Work out the finished part from the listing and answer in its coordinate system (mm). A direction names the side the tool comes from. Round coordinates to 2 decimals unless told otherwise and drop trailing zeros. Loops run counter-clockwise (first coordinate to the right, second up) from the corner with the lowest first, then second, coordinate; pieces in that order, holes last. Notation, with made-up numbers: M -12,76 L 8,76 A13 ccw 8,95 Z; hole C 43,33 d9. An arc over 180 degrees is marked long. One line per item, written item: value.
```python
from build123d import *

# Parameters (mm, degrees)
BOSS_EXTRUDE1_DEPTH = 6.35
CUT_EXTRUDE1_DEPTH  = 7.35
SKETCH3_R           = 2.286
CUT_EXTRUDE2_DEPTH  = 7.35
BOSS_EXTRUDE2_DEPTH = 6.35
SKETCH5_R           = 4.826
BOSS_EXTRUDE3_DEPTH = 6.35
SKETCH6_R           = 2.286
CUT_EXTRUDE3_DEPTH  = 13.7


with BuildPart() as part:
    # Sketch1 → Boss-Extrude1 (new body)
    with BuildSketch(Plane(origin=(0, 0, 0), x_dir=(1, 0, 0), z_dir=(0, 1, 0))):
        Polygon((0, 192.024), (6.35, 198.374), (196.85, 198.374), (203.2, 192.024), (203.2, 6.35), (196.85, 0), (6.35, 0), (0, 6.35), align=None)
    extrude(amount=BOSS_EXTRUDE1_DEPTH)

    # Sketch2 → Cut-Extrude1 (cut, through all)
    with BuildSketch(Plane(origin=(0, 6.35, 0), x_dir=(1, 0, 0), z_dir=(0, 1, 0))):
        with BuildLine():
            Line((45.682614691, 180.594), (152.691385309, 180.594))
            ThreePointArc((152.691385309, 180.594), (158.558020341, 176.674039796), (157.18151337, 169.753871939))
            Line((157.18151337, 169.753871939), (103.677128061, 116.24948663))
            ThreePointArc((103.677128061, 116.24948663), (99.187, 114.389614691), (94.696871939, 116.24948663))
            Line((94.696871939, 116.24948663), (41.19248663, 169.753871939))
            ThreePointArc((41.19248663, 169.753871939), (39.815979659, 176.674039796), (45.682614691, 180.594))
        make_face()
        with BuildLine():
            Line((17.78, 152.691385309), (17.78, 45.682614691))
            ThreePointArc((17.78, 45.682614691), (21.699960204, 39.815979659), (28.620128061, 41.19248663))
            Line((28.620128061, 41.19248663), (82.12451337, 94.696871939))
            ThreePointArc((82.12451337, 94.696871939), (83.984385309, 99.187), (82.12451337, 103.677128061))
            Line((82.12451337, 103.677128061), (28.620128061, 157.18151337))
            ThreePointArc((28.620128061, 157.18151337), (21.699960204, 158.558020341), (17.78, 152.691385309))
        make_face()
        with BuildLine():
            Line((45.682614691, 17.78), (152.691385309, 17.78))
            ThreePointArc((152.691385309, 17.78), (158.558020341, 21.699960204), (157.18151337, 28.620128061))
            Line((157.18151337, 28.620128061), (103.677128061, 82.12451337))
            ThreePointArc((103.677128061, 82.12451337), (99.187, 83.984385309), (94.696871939, 82.12451337))
            Line((94.696871939, 82.12451337), (41.19248663, 28.620128061))
            ThreePointArc((41.19248663, 28.620128061), (39.815979659, 21.699960204), (45.682614691, 17.78))
        make_face()
        with BuildLine():
            Line((185.42, 157.517385309), (185.42, 40.856614691))
            ThreePointArc((185.42, 40.856614691), (181.500039796, 34.989979659), (174.579871939, 36.36648663))
            Line((174.579871939, 36.36648663), (116.24948663, 94.696871939))
            ThreePointArc((116.24948663, 94.696871939), (114.389614691, 99.187), (116.24948663, 103.677128061))
            Line((116.24948663, 103.677128061), (174.579871939, 162.00751337))
            ThreePointArc((174.579871939, 162.00751337), (181.500039796, 163.384020341), (185.42, 157.517385309))
        make_face()
    extrude(amount=-CUT_EXTRUDE1_DEPTH, mode=Mode.SUBTRACT)

    # Sketch3 → Cut-Extrude2 (cut, through all)
    with BuildSketch(Plane(origin=(0, 6.35, 0), x_dir=(1, 0, 0), z_dir=(0, 1, 0))):
        with Locations((11.73734, 11.73734)):
            Circle(SKETCH3_R)
        with Locations((191.46266, 11.73734)):
            Circle(SKETCH3_R)
        with Locations((191.46266, 186.63666)):
            Circle(SKETCH3_R)
        with Locations((11.73734, 186.63666)):
            Circle(SKETCH3_R)
    extrude(amount=-CUT_EXTRUDE2_DEPTH, mode=Mode.SUBTRACT)

    # Sketch4 → Boss-Extrude2 (add)
    with BuildSketch(Plane(origin=(0, 6.35, 0), x_dir=(1, 0, 0), z_dir=(0, 1, 0))):
        with BuildLine():
            Line((111.554726315, 180.594), (91.645273685, 180.594))
            ThreePointArc((91.645273685, 180.594), (94.961453031, 179.659298195), (97.301368182, 177.130363636))
            ThreePointArc((97.301368182, 177.130363636), (101.6, 174.498), (105.898631818, 177.130363636))
            ThreePointArc((105.898631818, 177.130363636), (108.238546969, 179.659298195), (111.554726315, 180.594))
        make_face()
    extrude(amount=-BOSS_EXTRUDE2_DEPTH)

    # Sketch5 → Boss-Extrude3 (add)
    with BuildSketch(Plane.XZ):
        with Locations((101.6, -179.324)):
            Circle(SKETCH5_R)
    extrude(amount=BOSS_EXTRUDE3_DEPTH)

    # Sketch6 → Cut-Extrude3 (cut, through all)
    with BuildSketch(Plane.XZ.offset(6.35)):
        with Locations((101.6, -179.324)):
            Circle(SKETCH6_R)
        with Locations((92.71, -184.404)):
            Circle(SKETCH6_R)
        with Locations((110.49, -184.404)):
            Circle(SKETCH6_R)
    extrude(amount=-CUT_EXTRUDE3_DEPTH, mode=Mode.SUBTRACT)


solid = part.part
```
1) Find section B-B (x = 66). Give the vertices of the cut face in (y, z), then the cut area to 3 significant figures.
Check values:
outline: M 0,-198.37 L 6.35,-198.37 L 6.35,-180.59 L 0,-180.59 Z; M 0,-144.95 L 6.35,-144.95 L 6.35,-119.8 L 0,-119.8 Z; M 0,-78.57 L 6.35,-78.57 L 6.35,-53.43 L 0,-53.43 Z; M 0,-17.78 L 6.35,-17.78 L 6.35,0 L 0,0 Z
area: 545 mm2
2) The mould has two halves that part along X. Classify faces 1 (the face through (200.07, 3.13, -3.22)), 2 (the face through (103, 0, -101)), 3 (the face through (68.319, 3.219, -142.627)): +X half, -X half, draft (parallel to the pull), parting line (faces both ways), or undercut.
Check values:
face 1: +X half
face 2: draft
face 3: undercut
3) Find section C-C (x = 23). Give the vertices of the cut face in (y, z).
Check values:
outline: M 0,-198.37 L 6.35,-198.37 L 6.35,-158.94 L 0,-158.94 Z; M 0,-39.43 L 6.35,-39.43 L 6.35,0 L 0,0 Z
4) For faces 4 (the face through (17.78, 3, -100)), 5 (the face through (203.2, 3, -100)), determine the directions among +Z, -Z, +X, -X, +Y, -Y from which every point of the face is accessible in a straight line to the end or side of a thin tool.
Check values:
face 4: +Y, -Y
face 5: +Z, -Z, +X, +Y, -Y
5) Find the intervals of material crossed by probe 1 along Z at (x, y) = (110.49, 3.5); probe 2 along X at (y, z) = (5.5, -185.5); probe 3 along X at (y, z) = (3.25, -44), in increasing order. Write a range as from..to.
Check values:
probe 1: -198.37..-186.69, -182.12..-180.5, -123.06..-75.31, -17.78..0
probe 2: 0..9.75, 13.72..90.7, 94.72..108.48, 112.5..189.48, 193.45..203.2
probe 3: 0..18.01, 31.43..56.57, 141.8..166.95, 185.42..203.2
6) Find section A-A (z = -146.5). Give the vertices of the cut face in (x, y), then the cut area to 3 significant figures.
Check values:
outline: M 0,0 L 17.78,0 L 17.78,6.35 L 0,6.35 Z; M 39.3,0 L 64.45,0 L 64.45,6.35 L 39.3,6.35 Z; M 133.93,0 L 159.07,0 L 159.07,6.35 L 133.93,6.35 Z; M 185.42,0 L 203.2,0 L 203.2,6.35 L 185.42,6.35 Z
area: 545 mm2
7) Each of these flat-tipped pins is pushed along its axis until it touches: pin 1 (3 mm diameter, centred on x = 139, y = 3, fed in from +Z); pin 2 (4 mm diameter, centred on x = 11.74, z = -186.64, fed in from -Y); pin 3 (6 mm diameter, centred on x = 110.49, z = -184.404, fed in from -Y). Where does it stop, or does it pass through?
Check values:
pin 1: z = 0
pin 2: through
pin 3: y = 0
